Check sheet for the modelled part. Datum: model origin and axes. Units: mm. Face numbers are marked on the shaded views. A direction names the side the tool comes from. Coordinates: 2 decimals unless noted, no trailing zeros. Order: outer loops, then holes, each group sorted by start corner. A loop starts at its lowest first (then second) coordinate and runs counter-clockwise, first axis right, second up. Notation, with made-up numbers: M 33.5,39 L 79.5,39 A12 ccw 79.5,55 Z; hole C 17.5,83.5 d10. An arc over 180 degrees is marked long. Answer in a Markdown table with one row per item. Add a question column.
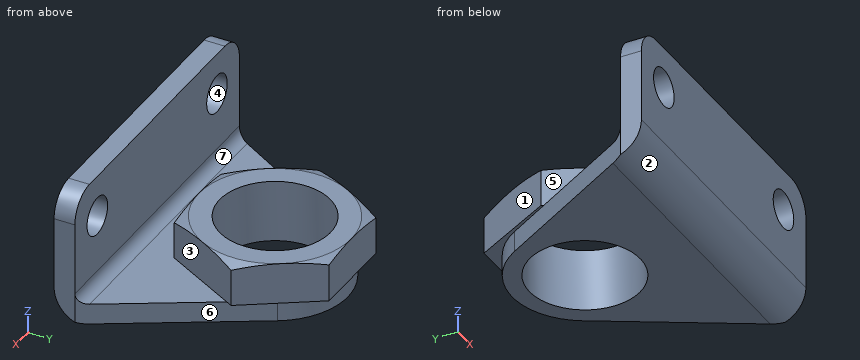
from build123d import *

# Parameters (mm, degrees)
EXTRUDE_START                   = -22
EXTRUDE_1_DEPTH                 = 44
CUT_EXTRUDE_1_DEPTH             = 10
CUT_EXTRUDE_1_DIRECTION_2_REACH = 42.869
SKETCH_6_R                      = 8
CUT_EXTRUDE_2_DEPTH             = 41.868692174
SKETCH_7_R                      = 2.75
CUT_EXTRUDE_3_DEPTH             = 41.015621949
FILLET_1_R                      = 3.9
EXTRUDE_2_DEPTH                 = 6
SKETCH_11_R                     = 8
CUT_EXTRUDE_4_DEPTH             = 42.243181255


with BuildPart() as part:
    # 草图4 → 凸台-拉伸1 (new body)
    with BuildSketch(Plane(origin=(0, 0, 0), x_dir=(0, 0, -1), z_dir=(1, 0, 0)).offset(EXTRUDE_START)):
        with BuildLine():
            Line((-19, 0), (-4.625, 0))
            ThreePointArc((-4.625, 0), (-1.354631137, 1.354631137), (0, 4.625))
            Line((0, 4.625), (0, 30.5))
            Line((0, 30.5), (-3, 30.5))
            Line((-3, 30.5), (-3, 4.625))
            ThreePointArc((-3, 4.625), (-3.475951481, 3.475951481), (-4.625, 3))
            Line((-4.625, 3), (-19, 3))
            Line((-19, 3), (-19, 0))
        make_face()
    extrude(amount=EXTRUDE_1_DEPTH)

    # 草图5 → 切除-拉伸1 (cut)
    with BuildSketch(Plane.XY.offset(3)):
        with BuildLine():
            Line((-9.082524892, 25.268561625), (-22, 3))
            Line((-22, 3), (-22, 31.5))
            Line((-22, 31.5), (22, 31.5))
            Line((22, 31.5), (22, 3))
            Line((22, 3), (9.082524892, 25.268561625))
            ThreePointArc((9.082524892, 25.268561625), (0, 30.5), (-9.082524892, 25.268561625))
        make_face()
    extrude(amount=-CUT_EXTRUDE_1_DEPTH, mode=Mode.SUBTRACT)

    # 切除-拉伸1 direction 2: up to this face of the body (flat: up to its plane)
    cut_extrude_1_direction_2_end = Plane(part.part.faces().sort_by_distance((0, 1.5, 19))[0])
    # 草图5 → 切除-拉伸1 direction 2 (cut, up to the picked face)
    with BuildSketch(Plane.XY.offset(3), mode=Mode.PRIVATE) as cut_extrude_1_direction_2_sk1:
        with BuildLine():
            Line((-9.082524892, 25.268561625), (-22, 3))
            Line((-22, 3), (-22, 31.5))
            Line((-22, 31.5), (22, 31.5))
            Line((22, 31.5), (22, 3))
            Line((22, 3), (9.082524892, 25.268561625))
            ThreePointArc((9.082524892, 25.268561625), (0, 30.5), (-9.082524892, 25.268561625))
        make_face()
    cut_extrude_1_direction_2_tool1 = split(extrude(cut_extrude_1_direction_2_sk1.sketch, amount=CUT_EXTRUDE_1_DIRECTION_2_REACH, mode=Mode.PRIVATE), bisect_by=cut_extrude_1_direction_2_end, keep=Keep.BOTH, mode=Mode.PRIVATE)
    add(cut_extrude_1_direction_2_tool1.solids().sort_by(Axis((-15.994729, 14.397326, 3), (0, 0, 1)))[0], mode=Mode.SUBTRACT)

    # 草图6 → 切除-拉伸2 (cut, through all)
    with BuildSketch(Plane.XY.offset(3)):
        with Locations((0, 20)):
            Circle(SKETCH_6_R)
    extrude(amount=-CUT_EXTRUDE_2_DEPTH, mode=Mode.SUBTRACT)

    # 草图7 → 切除-拉伸3 (cut, through all)
    with BuildSketch(Plane(origin=(0, 3, 0), x_dir=(1, 0, 0), z_dir=(0, 1, 0))):
        with Locations(Location((16, -13, 0), (0, 0, 270))):
            Circle(SKETCH_7_R)
        with Locations(Location((-16, -13, 0), (0, 0, 90))):
            Circle(SKETCH_7_R)
    extrude(amount=-CUT_EXTRUDE_3_DEPTH, mode=Mode.SUBTRACT)

    # 圆角1
    fillet_1_edges = [part.edges().sort_by_distance(p)[0] for p in [
        (-22, 1.5, 19),
        (22, 1.5, 19),
    ]]
    fillet(fillet_1_edges, radius=FILLET_1_R)

    # 草图9 → 凸台-拉伸2 (add)
    with BuildSketch(Plane.XY.offset(3)):
        Polygon((-5.937171044, 9), (6.562828956, 9), (12.797171044, 20.550578963), (5.937171044, 31), (-6.562828956, 31), (-12.797171044, 19.449421037), align=None)
    extrude(amount=EXTRUDE_2_DEPTH)

    # 草图10 → 切除-旋转1 (revolve, cut)
    with BuildSketch(Plane(origin=(0, 0, 0), x_dir=(0, 0, 1), z_dir=(1, 0, 0))):
        Polygon((9, -31), (9, -34.5), (7.72610418, -34.5), align=None)
    revolve(axis=Axis((0, 20, 71.423754158), (0, 0, -1)), mode=Mode.SUBTRACT)

    # 草图11 → 切除-拉伸4 (cut, through all)
    with BuildSketch(Plane(origin=(0, 0, 3), x_dir=(-1, 0, 0), z_dir=(0, 0, -1))):
        with Locations(Location((0, 20, 0), (0, 0, 180))):
            Circle(SKETCH_11_R)
    extrude(amount=-CUT_EXTRUDE_4_DEPTH, mode=Mode.SUBTRACT)


solid = part.part
1. Set-up check for the marked faces 5, 6 and 7: record each of +Z, -Z, +X, -X, +Y, -Y from which the full face is reachable in a straight line by a thin tool's end or side.
2. Scan lines: line 1 (X direction, y = 1.4, z = 13); line 2 (Y direction, x = 0, z = 6.25); line 3 (Y direction, x = -6, z = 6). Record each from-to range of solid material in increasing order.
3. Section check C-C on y = 2. Enter the section's corners in (x, z).
4. Section check B-B on z = 13. Enter the section's corners in (x, y).
5. Go/stop test with flat-tipped pins: pin 1 Ø10 at (x, z) = (14, 16.5) entering from +Y; pin 2 Ø8 at (y, z) = (12.5, 2.5) entering from +X; pin 3 Ø17.5 at (x, y) = (-5.5, 15) entering from +Z; pin 4 Ø3.5 at (x, z) = (-16, 13) entering from -Y. Record where each tip stops, or that it passes through.
6. Section check D-D on z = 1.5. Enter the section's corners in (x, y), then the cut area to 3 significant figures.
7. Release check for a two-part mould opening along X. For the marked faces 1, 2, 3 and 4 record: released by +X, released by -X, zero draft, split by the parting line, or undercut.
Result sheet:
| question | item | result |
|---|---|---|
| 1 | face 5 | +Z, -X |
| 1 | face 6 | -Z, +X, +Y |
| 1 | face 7 | +Z, +X, -X |
| 2 | line 1 | -22 to -18.75, -13.25 to 13.25, 18.75 to 22 |
| 2 | line 2 | 0 to 3, 9 to 12, 28 to 31 |
| 2 | line 3 | 0 to 3, 9.1 to 14.71, 25.29 to 31 |
| 3 | outline | M -22,0.82 L 22,0.82 L 22,15.1 A3.9 ccw 18.1,19 L -18.1,19 A3.9 ccw -22,15.1 Z; hole C -16,13 d5.5; hole C 16,13 d5.5 |
| 4 | outline | M -22,0 L -18.75,0 L -18.75,3 L -22,3 Z; M -13.25,0 L 13.25,0 L 13.25,3 L -13.25,3 Z; M 18.75,0 L 22,0 L 22,3 L 18.75,3 Z |
| 5 | pin 1 | y = 3 |
| 5 | pin 2 | x = 18.81 |
| 5 | pin 3 | z = 9 |
| 5 | pin 4 | through |
| 6 | outline | M -22,1.22 L 22,1.22 L 22,3 L 9.08,25.27 A10.5 ccw -9.08,25.27 L -22,3 Z; hole C 0,20 d16 |
| 6 | area | 637 mm^2 |
| 7 | face 1 | released by -X |
| 7 | face 2 | zero draft |
| 7 | face 3 | released by +X |
| 7 | face 4 | undercut |
